from build123d import *


with BuildPart() as part:
    # Profile Sketch → Profile Revolve (revolve)
    with BuildSketch(Plane(origin=(0, 0, 0), x_dir=(0, 0, -1), z_dir=(1, 0, 0)), mode=Mode.PRIVATE) as profile_revolve_sk:
        Polygon((-6, -3.499999985), (-6, -5.087499985), (-11, -5.087499985), (-14.175, -5.087499985), (-14.175, -1.585), (-17.375, -1.585), (-17.375, 1.585), (-14.175, 1.585), (-14.175, 5.087499985), (-11, 5.087499985), (-11, -3.499999985), align=None)
    revolve(profile_revolve_sk.sketch.rotate(Axis((0, -5.087499985, 0), (0, 1, 0)), 180), axis=Axis((0, -5.087499985, 0), (0, 1, 0)))


solid = part.part
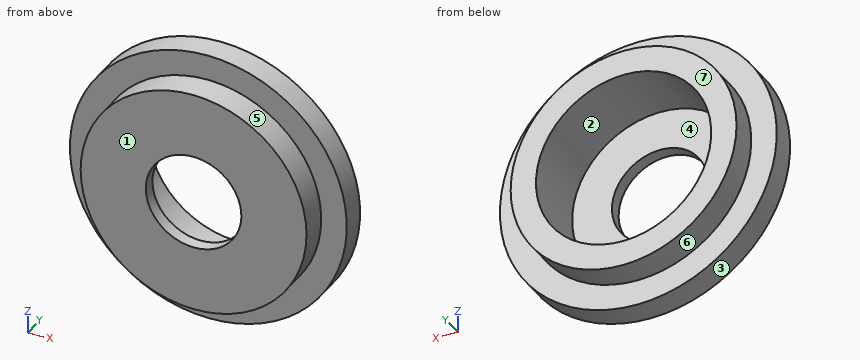
Check sheet for the modelled part. Datum: model origin and axes. Units: mm. Face numbers are marked on the shaded views. A direction names the side the tool comes from. Give positions to 0.01 mm unless a question says otherwise; leave off trailing zeros. Loops run counter-clockwise (first coordinate to the right, second up) from the corner with the lowest first, then second, coordinate; pieces in that order, holes last. Notation, with made-up numbers: M 39.25,46.25 L 53.25,46.25 A19 cw 53.25,73.25 Z; hole C 75,-4 d9. An arc over 180 degrees is marked long. Return JSON: item names as keys, results as strings. Group by question number.
1. Cross-section at C-C on y = 4. Record the boundary of the cut face in (x, z) (3 decimals), plus the area to 3 significant figures.
2. Tool access check on the marked faces 5, 6 and 7. Record the directions out of +Z, -Z, +X, -X, +Y, -Y that give a thin tool (end or side, any length) a straight path to the whole face; none if there is none.
3. Cross-section at A-A on x = 0. Record the boundary of the cut face in (y, z) (1 decimal), plus the area to 3 significant figures.
4. Cross-section at B-B on z = -5. Record the boundary of the cut face in (x, y) (1 decimal).
5. Go/stop test with flat-tipped pins: pin 1 (1 mm diameter, centred on y = -4, z = 9, fed in from +X); pin 2 (19 mm diameter, centred on x = 0, z = 0, fed in from -Y); pin 3 (1.5 mm diameter, centred on x = 14, y = 1.5, fed in from -Z); pin 4 (1.5 mm diameter, centred on x = -4.5, z = -8, fed in from +Y). Record where each tip stops, or that it passes through.
6. Cross-section at D-D on z = -9. Record the boundary of the cut face in (x, y) (1 decimal), plus the area to 3 significant figures.
7. Thickness scan on L1, parallel to X at y = -1, z = 0 (3 decimals); L2, parallel to X at y = -4, z = 0 (3 decimals); L3, parallel to Z at x = -1, y = 3. Record the ranges inside material, lowest first.
8. Mould release check, pull along Z, two halves, no side actions. Record for the marked faces 1, 2, 3 and 4: released by +Z, released by -Z, zero draft, split by the parting line, or undercut.
Return value:
{
 "1": {"outline": "C 0,0 d28.35; hole C 0,0 d22", "area": "251 mm^2"},
 "2": {"face 5": "-Y", "face 6": "+Y", "face 7": "+Z, -Z, +X, -X, +Y"},
 "3": {"outline": "M -5.1,-14.2 L -1.6,-14.2 L -1.6,-17.4 L 1.6,-17.4 L 1.6,-14.2 L 5.1,-14.2 L 5.1,-11 L -3.5,-11 L -3.5,-6 L -5.1,-6 Z; M -5.1,6 L -3.5,6 L -3.5,11 L 5.1,11 L 5.1,14.2 L 1.6,14.2 L 1.6,17.4 L -1.6,17.4 L -1.6,14.2 L -5.1,14.2 Z", "area": "101 mm^2"},
 "4": {"outline": "M -16.6,-1.6 L -13.3,-1.6 L -13.3,-5.1 L -3.3,-5.1 L -3.3,-3.5 L -9.8,-3.5 L -9.8,5.1 L -13.3,5.1 L -13.3,1.6 L -16.6,1.6 Z; M 3.3,-5.1 L 13.3,-5.1 L 13.3,-1.6 L 16.6,-1.6 L 16.6,1.6 L 13.3,1.6 L 13.3,5.1 L 9.8,5.1 L 9.8,-3.5 L 3.3,-3.5 Z"},
 "5": {"pin 1": "x = 11.34", "pin 2": "y = -5.09", "pin 3": "z = -11.24", "pin 4": "y = -3.5"},
 "6": {"outline": "M -14.9,-1.6 L -11,-1.6 L -11,-5.1 L 11,-5.1 L 11,-1.6 L 14.9,-1.6 L 14.9,1.6 L 11,1.6 L 11,5.1 L 6.3,5.1 L 6.3,-3.5 L -6.3,-3.5 L -6.3,5.1 L -11,5.1 L -11,1.6 L -14.9,1.6 Z", "area": "139 mm^2"},
 "7": {"L1": "-17.375 to -11, 11 to 17.375", "L2": "-14.175 to -6, 6 to 14.175", "L3": "-14.14 to -10.95, 10.95 to 14.14"},
 "8": {"face 1": "zero draft", "face 2": "undercut", "face 3": "split by the parting line", "face 4": "undercut"}
}
